Can you work these out from the model? Positions are in its coordinate system, mm. Face numbers are marked on the shaded views. Give positions to 0.01 mm unless a question says otherwise; leave off trailing zeros. Loops run counter-clockwise (first coordinate to the right, second up) from the corner with the lowest first, then second, coordinate; pieces in that order, holes last.
from build123d import *

# Parameters (mm, degrees)
F0_R     = 17.1577
F0_R_2   = 2.38
F0_R_3   = 1.47
F1_DEPTH = 4
F2_R     = 1.47
F3_DEPTH = 2.37


with BuildPart() as f1:
    # F0 (on Top) → F1 (new body)
    with BuildSketch(Plane.XY):
        Circle(F0_R)
        with Locations((-8.64629, -8.64629)):
            Circle(F0_R_2, mode=Mode.SUBTRACT)
        with Locations((0, -9.7077)):
            Circle(F0_R_2, mode=Mode.SUBTRACT)
        with Locations((8.64629, -8.64629)):
            Circle(F0_R_2, mode=Mode.SUBTRACT)
        with Locations((-9.7077, 0)):
            Circle(F0_R_2, mode=Mode.SUBTRACT)
        with Locations((-8.64629, 8.64629)):
            Circle(F0_R_2, mode=Mode.SUBTRACT)
        Circle(F0_R_3, mode=Mode.SUBTRACT)
        with Locations((9.7077, 0)):
            Circle(F0_R_2, mode=Mode.SUBTRACT)
        with Locations((0, 9.7077)):
            Circle(F0_R_2, mode=Mode.SUBTRACT)
        with Locations((8.64629, 8.64629)):
            Circle(F0_R_2, mode=Mode.SUBTRACT)
    extrude(amount=F1_DEPTH)

    # F2 (on face) → F3 (cut)
    with BuildSketch(Plane.XY.offset(4)):
        Polygon((3.117599, 0.024062), (1.537961, 2.71195), (-1.579637, 2.687889), (-3.117599, -0.024062), (-1.537961, -2.71195), (1.579637, -2.687889), align=None)
        Circle(F2_R, mode=Mode.SUBTRACT)
    extrude(amount=-F3_DEPTH, mode=Mode.SUBTRACT)


solid = f1.part
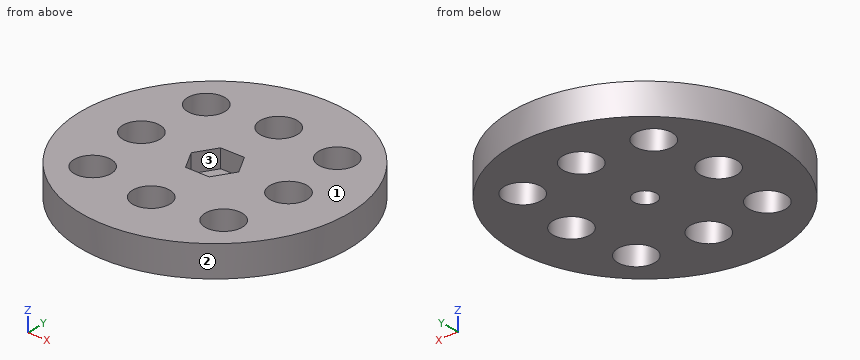
(1) Will these pins go through, and if not, where does the flat tip stop? P1, Ø1, axis at x = 8, z = 2, coming from the +Y side; P2, Ø4.5, axis at x = 0, y = 0, coming from the +Z side; P3, Ø1.5, axis at x = 9, z = 3, coming from the +Y side.
Returned:
P1: stops at y = 15.43
P2: stops at z = 1.63
P3: stops at y = 15.04
(2) Suppose I cut it at D-D on y = 14. List the corners of the cut face in (x, z) for me, plus the area to 3 significant figures.
Returned:
outline: (-9.92, 0) - (9.92, 0) - (9.92, 4) - (-9.92, 4) - close
area: 79.4 mm2
(3) Suppose I cut it at B-B on z = 0.5. Give the number of separate pieces and of enclosed holes in the cut face, plus the area to 3 significant figures.
Returned:
separate pieces: 1
enclosed holes: 9
area: 776 mm2
(4) Please list where these lines run through material, in increasing order: probe 1 along Y at (x, z) = (6.5, 2); probe 2 along X at (y, z) = (-0.5, 3.05); probe 3 along Y at (x, z) = (-10, 0.6).
Returned:
probe 1: y = -15.88 to -9.67, -7.62 to 7.62, 9.67 to 15.88
probe 2: x = -17.15 to -12.03, -7.38 to -2.84, 2.82 to 7.38, 12.03 to 17.15
probe 3: y = -13.94 to -10.6, -6.69 to -2.36, 2.36 to 6.69, 10.6 to 13.94
(5) Suppose I cut it at A-A on x = 0. List the corners of the cut face in (y, z) for me.
Returned:
outline: (-17.16, 0) - (-12.09, 0) - (-12.09, 4) - (-17.16, 4) - close; (-7.33, 0) - (-1.47, 0) - (-1.47, 1.63) - (-2.7, 1.63) - (-2.7, 4) - (-7.33, 4) - close; (1.47, 0) - (7.33, 0) - (7.33, 4) - (2.7, 4) - (2.7, 1.63) - (1.47, 1.63) - close; (12.09, 0) - (17.16, 0) - (17.16, 4) - (12.09, 4) - close
(6) Suppose I cut it at C-C on x = 5. List the corners of the cut face in (y, z) for me, plus the area to 3 significant figures.
Returned:
outline: (-16.41, 0) - (16.41, 0) - (16.41, 4) - (-16.41, 4) - close
area: 131 mm2
(7) Thinking about a two-plate mould opening in Y: for the marked faces 1, 2 and 3, which applies, pulls with the +Y half, pulls with the -Y half, needs draft (parallel to the pull), parting line crosses it, or undercut?
Returned:
face 1: needs draft
face 2: parting line crosses it
face 3: undercut
